Verification items for the finished model (mm, model axes). Face numbers are marked on the shaded views. A direction names the side the tool comes from. Give positions to 0.01 mm unless a question says otherwise; leave off trailing zeros. Loops run counter-clockwise (first coordinate to the right, second up) from the corner with the lowest first, then second, coordinate; pieces in that order, holes last. Notation, with made-up numbers: M -26.75,21 L -11.75,21 A10 cw -11.75,39 Z; hole C 51,25.5 d2. An arc over 180 degrees is marked long. Answer in a Markdown table with one row per item.
```python
from build123d import *

# Parameters (mm, degrees)
PAD_DEPTH       = 35
SKETCH001_R     = 16.5
POCKET_DEPTH    = 5
POCKET001_DEPTH = 5
FILLET_R        = 1
FILLET001_R     = 5
SKETCH003_R     = 2.6
POCKET002_DEPTH = 5
SKETCH004_W     = 36
SKETCH004_H     = 3
PAD001_DEPTH    = 19
FILLET002_R     = 2
FILLET003_R     = 2
FILLET004_R     = 1


with BuildPart() as part:
    # Sketch → Pad (new body, symmetric)
    with BuildSketch(Plane.YZ):
        Polygon((34.3, -18), (34.3, -21), (-16.5, -21), (-16.5, 21), (12.5, 21), (12.5, 18), (-12.5, 18), (-12.5, -18), align=None)
    extrude(amount=PAD_DEPTH, both=True)

    # Sketch001 (on Face3 of Pad) → Pocket (cut)
    with BuildSketch(Plane(origin=(0, -16.5, 0), x_dir=(0, 0, -1), z_dir=(0, -1, 0))):
        with Locations((0, 33)):
            Circle(SKETCH001_R)
        with Locations((0, -33)):
            Circle(SKETCH001_R)
        with BuildLine():
            ThreePointArc((-8.5, 8), (-16.5, 0), (-8.5, -8))
            Line((-8.5, -8), (8.5, -8))
            ThreePointArc((8.5, -8), (16.5, 0), (8.5, 8))
            Line((-8.5, 8), (8.5, 8))
        make_face()
    extrude(amount=-POCKET_DEPTH, mode=Mode.SUBTRACT)

    # Sketch002 (on Face3 of Pocket) → Pocket001 (cut)
    with BuildSketch(Plane.YX.offset(21)):
        with BuildLine():
            ThreePointArc((-6.5, -22.2), (-9.7, -25.4), (-6.5, -28.6))
            Line((-6.5, -28.6), (26.5, -28.6))
            ThreePointArc((26.5, -28.6), (29.7, -25.4), (26.5, -22.2))
            Line((-6.5, -22.2), (26.5, -22.2))
        make_face()
        with BuildLine():
            ThreePointArc((-6.5, 28.6), (-9.7, 25.4), (-6.5, 22.2))
            Line((-6.5, 22.2), (26.5, 22.2))
            ThreePointArc((26.5, 22.2), (29.7, 25.4), (26.5, 28.6))
            Line((-6.5, 28.6), (26.5, 28.6))
        make_face()
        with BuildLine():
            ThreePointArc((-3.306398, 8), (-9.7, 0), (-3.306398, -8))
            Line((-3.306398, -8), (34.3, -16.5))
            ThreePointArc((34.3, -16.5), (54.94564, 0), (34.3, 16.5))
            Line((-3.306398, 8), (34.3, 16.5))
        make_face()
    extrude(amount=-POCKET001_DEPTH, mode=Mode.SUBTRACT)

    # Fillet
    fillet_edges = [part.edges().sort_by_distance(p)[0] for p in [
        (35, -14.5, 16.378339),
        (-35, -14.5, 16.378339),
        (-35, -14.5, -16.378339),
        (35, -14.5, -16.378339),
    ]]
    fillet(fillet_edges, radius=FILLET_R)

    # Fillet001
    fillet001_edges = [part.edges().sort_by_distance(p)[0] for p in [
        (35, 34.3, -19.5),
        (16.5, 34.3, -19.5),
        (-16.5, 34.3, -19.5),
        (-35, 34.3, -19.5),
    ]]
    fillet(fillet001_edges, radius=FILLET001_R)

    # Sketch003 (on Face39 of Fillet001) → Pocket002 (cut)
    with BuildSketch(Plane(origin=(0, 0, 21), x_dir=(0, -1, 0), z_dir=(0, 0, 1))):
        with Locations((0, 20)):
            Circle(SKETCH003_R)
        with Locations((0, -20)):
            Circle(SKETCH003_R)
    extrude(amount=-POCKET002_DEPTH, mode=Mode.SUBTRACT)

    # Sketch004 (on Face4 of Pocket002) → Pad001 (join)
    with BuildSketch(Plane.ZX.offset(-12.5)):
        with Locations((0, -12.619025)):
            Rectangle(SKETCH004_W, SKETCH004_H)
        with Locations((0, 12.619025)):
            Rectangle(SKETCH004_W, SKETCH004_H)
    extrude(amount=PAD001_DEPTH)

    # Fillet002
    fillet002_edges = [part.edges().sort_by_distance(p)[0] for p in [
        (14.119025, -12.5, 0),
        (-11.119025, -12.5, 0),
        (11.119025, -12.5, 0),
        (-14.119025, -12.5, 0),
    ]]
    fillet(fillet002_edges, radius=FILLET002_R)

    # Fillet003
    fillet003_edges = [part.edges().sort_by_distance(p)[0] for p in [
        (-25.559513, -12.5, 18),
        (0, -12.5, 18),
        (25.559513, -12.5, 18),
    ]]
    fillet(fillet003_edges, radius=FILLET003_R)

    # Fillet004
    fillet004_edges = [part.edges().sort_by_distance(p)[0] for p in [
        (25.559513, -12.5, -18),
        (-25.559513, -12.5, -18),
    ]]
    fillet(fillet004_edges, radius=FILLET004_R)


solid = part.part
```
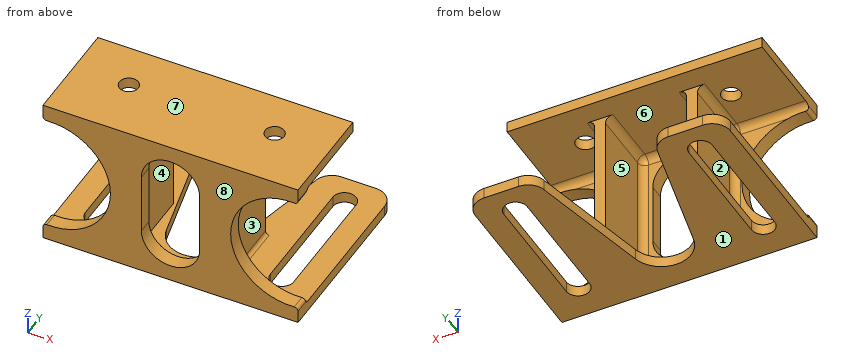
Item 1: Go/stop test with flat-tipped pins: pin 1 (3 mm diameter, centred on y = -14.5, z = -2, fed in from +X); pin 2 (5 mm diameter, centred on x = -28, y = 20.5, fed in from +Z); pin 3 (0.9 mm diameter, centred on x = 13, z = 19.5, fed in from +Y). Record where each tip stops, or that it passes through.
Reported:
| item | result |
|---|---|
| pin 1 | stops at x = 16.88 |
| pin 2 | stops at z = -18 |
| pin 3 | stops at y = 12.5 |
Item 2: Release check for a two-part mould opening along Z. For the marked faces 5, 6, 7 and 8 record: released by +Z, released by -Z, zero draft, split by the parting line, or undercut.
Reported:
| item | result |
|---|---|
| face 5 | undercut |
| face 6 | undercut |
| face 7 | released by +Z |
| face 8 | zero draft |
Item 3: Sectioned sample at D-D (x = -25.4). Record the cut outline in (y, z).
Reported:
| item | result |
|---|---|
| outline | M -16.5,-21 L -9.7,-21 L -9.7,-18 L -11.5,-18 A1 cw -12.5,-17 L -12.5,-14.65 L -16.5,-14.65 Z; M -16.5,14.65 L -12.5,14.65 L -12.5,16 A2 cw -10.5,18 L 12.5,18 L 12.5,21 L -16.5,21 Z; M 29.7,-21 L 34.3,-21 L 34.3,-18 L 29.7,-18 Z |
Item 4: Scan lines: L1, parallel to X at y = 0, z = 19; L2, parallel to X at y = -14, z = -0.5; L3, parallel to X at y = 4, z = -17. Record each from-to range of solid material in increasing order. Write a range as [from, to].
Reported:
| item | result |
|---|---|
| L1 | x = [-35, -22.6], [-17.4, 17.4], [22.6, 35] |
| L2 | x = [-16.51, -8], [8, 16.51] |
| L3 | x = [-14.12, -11.12], [11.12, 14.12] |
Item 5: Sectioned sample at C-C (y = -7.5). State how many separate pieces and enclosed holes the cut face has, and give its area (3 significant figures).
Reported:
| item | result |
|---|---|
| separate pieces | 3 |
| enclosed holes | 0 |
| area | 570 mm^2 |
Item 6: Sectioned sample at A-A (x = 33). Record the cut outline in (y, z).
Reported:
| item | result |
|---|---|
| outline | M -16.5,-21 L 33.3,-21 L 33.3,-18 L -11.5,-18 A1 cw -12.5,-17 L -12.5,-16.5 L -16.5,-16.5 Z; M -16.5,16.5 L -12.44,16.5 A2 cw -10.5,18 L 12.5,18 L 12.5,21 L -16.5,21 Z |
Item 7: Sectioned sample at B-B (z = 2). Record the cut outline in (x, y), and give its area (3 significant figures).
Reported:
| item | result |
|---|---|
| outline | M -16.62,-16.5 L -8,-16.5 L -8,-12.5 L -9.12,-12.5 A2 cw -11.12,-10.5 L -11.12,6.5 L -14.12,6.5 L -14.12,-10.5 A2 cw -16.12,-12.5 L -16.62,-12.5 Z; M 8,-16.5 L 16.62,-16.5 L 16.62,-12.5 L 16.12,-12.5 A2 cw 14.12,-10.5 L 14.12,6.5 L 11.12,6.5 L 11.12,-10.5 A2 cw 9.12,-12.5 L 8,-12.5 Z |
| area | 186 mm^2 |
Item 8: Tool access check on the marked faces 1, 2, 3 and 4. Record the directions out of +Z, -Z, +X, -X, +Y, -Y that give a thin tool (end or side, any length) a straight path to the whole face; none if there is none.
Reported:
| item | result |
|---|---|
| face 1 | -Z, +X, -X, +Y, -Y |
| face 2 | -X, +Y |
| face 3 | +X, +Y |
| face 4 | +Y |
